Geometry check sheet. Reference: drawing and pictorial views, mm from the part's lowest x, y, z. A direction names the side the tool comes from. Give positions to 0.01 mm unless a question says otherwise; leave off trailing zeros. Loops run counter-clockwise (first coordinate to the right, second up) from the corner with the lowest first, then second, coordinate; pieces in that order, holes last. Notation, with made-up numbers: (26, -33) - (77, -33) arc R21 ccw to (77, 6) - close; hole circle Ø8 at (-6.75, 51.5). An arc over 180 degrees is marked (long way). Answer in a Markdown table with one row per item. Add a question column.
(1) Thickness scan on L1, parallel to Y at x = 4, z = 2.1; L2, parallel to Z at x = 4.75, y = 0.95; L3, parallel to Y at x = 7.5, z = 3.45. Record the ranges inside material, lowest first.
(2) Draft check along Z on the marked faces 1, 2 and 3. Enter one of: released by +Z, released by -Z, zero draft, split by the parting line, or undercut.
(3) Go/stop test with flat-tipped pins: P1, Ø1.6, axis at x = 7, y = 3, coming from the +Z side; P2, Ø1.5, axis at x = 6.5, z = 3, coming from the -Y side. Record where each tip stops, or that it passes through.
(4) Set-up check for the marked faces 4 and 5: record each of +Z, -Z, +X, -X, +Y, -Y from which the full face is reachable in a straight line by a thin tool's end or side.
(5) Sectioned sample at C-C on z = 2. Enter the section's corners in (x, y) (3 decimals).
(6) Sectioned sample at A-A on x = 6.75. Enter the section's corners in (y, z), then the cut area to 3 significant figures.
(7) Sectioned sample at D-D on x = 2.5. Enter the section's corners in (y, z), then the cut area to 3 significant figures.
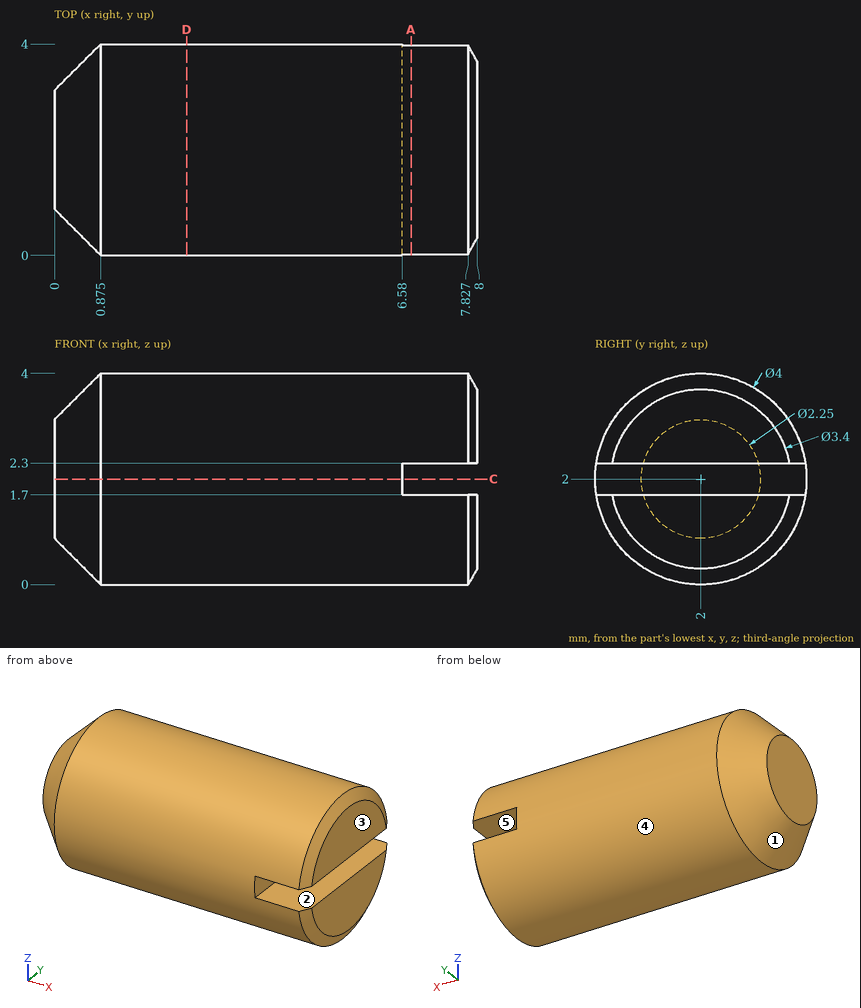
Reply:
| question | item | result |
|---|---|---|
| 1 | L1 | 0 to 4 |
| 1 | L2 | 0.3 to 3.7 |
| 1 | L3 | 0.62 to 3.38 |
| 2 | face 1 | split by the parting line |
| 2 | face 2 | undercut |
| 2 | face 3 | zero draft |
| 3 | P1 | z = 3.99 |
| 3 | P2 | y = 0.02 |
| 4 | face 4 | +X, -X |
| 4 | face 5 | +X, +Y, -Y |
| 5 | outline | (0, 0.875) - (0.875, 0) - (6.58, 0) - (6.58, 4) - (0.875, 4) - (0, 3.125) - close |
| 6 | outline | (0.02, 1.7) arc R2 ccw to (3.98, 1.7) - close; (0.02, 2.3) - (3.98, 2.3) arc R2 ccw to start |
| 6 | area | 10.2 mm^2 |
| 7 | outline | circle Ø4 at (2, 2) |
| 7 | area | 12.6 mm^2 |
